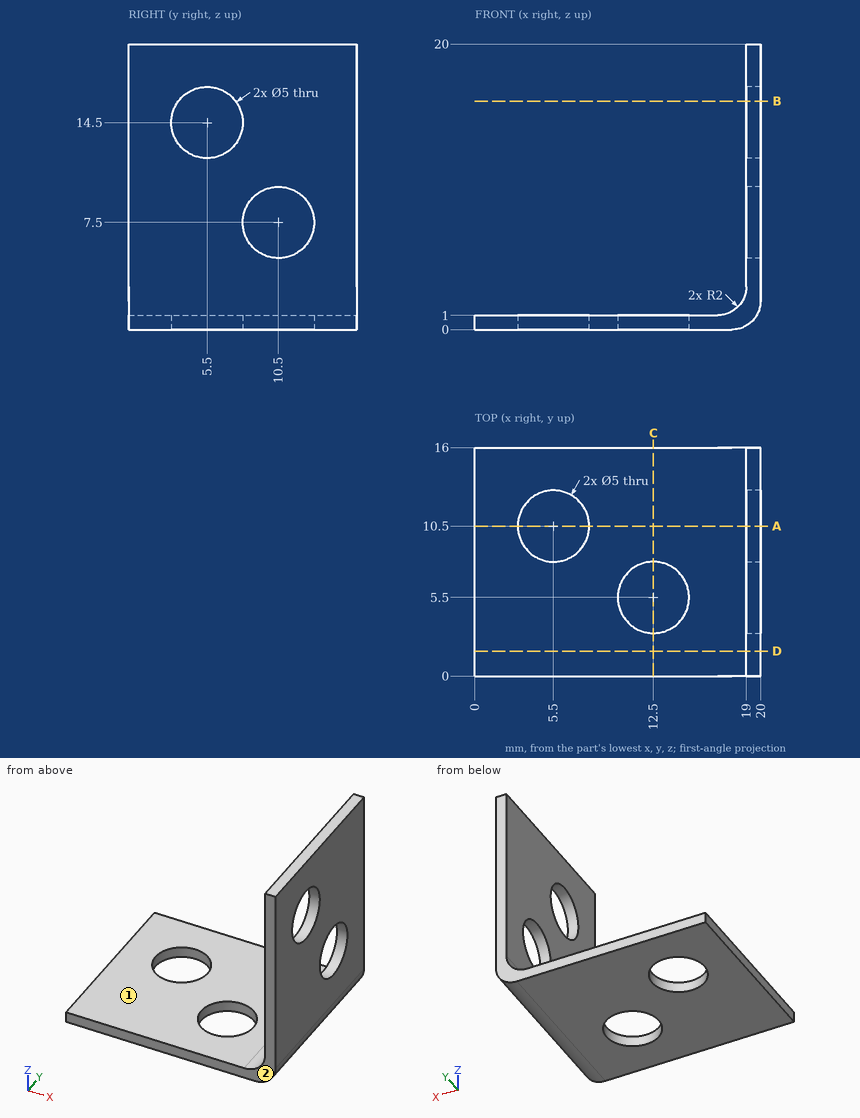
Here's the drawing with two shaded views (mm, measured from the low corner). I have some questions. A direction names the side the tool comes from. Coordinates: 2 decimals unless noted, no trailing zeros. Write each loop counter-clockwise with the first axis right and the second up, starting at its lowest first coordinate (ties: lowest second). Pieces come first, ordered by that corner, then holes. Notation, with made-up numbers: (89, -12.75) -> (145, -12.75) arc R16 cw to (145, 10.25) -> close; hole circle Ø11 at (-2, -13.75). An arc over 180 degrees is marked (long way). One line per question, with ' | ' between items. Start each with the question number.
1. If we section it at B-B (z = 16): Please give me the cut outline in (x, y), and give its area (3 significant figures).
2. Will these pins go through, and if not, where does the flat tip stop? P1, Ø8, axis at y = 9, z = 10, coming from the -X side; P2, Ø10, axis at x = 2.5, z = 8, coming from the +Y side; P3, Ø1.5, axis at x = 17, y = 7.5, coming from the +Z side.
3. If we section it at C-C (x = 12.5): Please give me the cut outline in (y, z), and give its area (3 significant figures).
4. Please list where these lines run through material, in increasing order: line 1 along Y through (x, z) = (12.5, 0.5); line 2 along Y through (x, z) = (5.5, 0.35); line 3 along X through (y, z) = (13, 17.5).
5. If we section it at A-A (y = 10.5): Please give me the cut outline in (x, z).
6. If we section it at D-D (y = 1.75): Please give me the cut outline in (x, z), and give its area (3 significant figures).
7. For the marked faces 1 and 2, which set-ups out of +Z, -Z, +X, -X, +Y, -Y let a thin tool reach every point of the face, with its end or its side?
Return value:
1) outline: (19, 0) -> (20, 0) -> (20, 3.5) -> (19, 3.5) -> close; (19, 7.5) -> (20, 7.5) -> (20, 16) -> (19, 16) -> close | area: 12.0 mm²
2) P1: stops at x = 19 | P2: passes through | P3: stops at z = 1.15
3) outline: (0, 0) -> (3, 0) -> (3, 1) -> (0, 1) -> close; (8, 0) -> (16, 0) -> (16, 1) -> (8, 1) -> close | area: 11.0 mm²
4) line 1: y = 0 to 3, 8 to 16 | line 2: y = 0 to 8, 13 to 16 | line 3: x = 19 to 20
5) outline: (0, 0) -> (3, 0) -> (3, 1) -> (0, 1) -> close; (8, 0) -> (18, 0) arc R2 ccw to (20, 2) -> (20, 5) -> (19, 5) -> (19, 3) arc R2 cw to (17, 1) -> (8, 1) -> close; (19, 10) -> (20, 10) -> (20, 20) -> (19, 20) -> close
6) outline: (0, 0) -> (18, 0) arc R2 ccw to (20, 2) -> (20, 20) -> (19, 20) -> (19, 3) arc R2 cw to (17, 1) -> (0, 1) -> close | area: 39.0 mm²
7) face 1: +Z, -X, +Y, -Y | face 2: +Z, -Z, +X, -X, -Y
